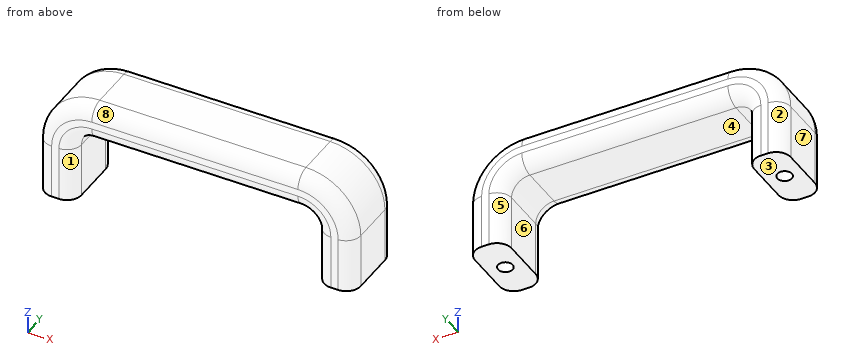
from build123d import *

# Parameters (mm, degrees)
F1_DEPTH = 25.4
F2_R     = 5.08
F3_R     = 2.54
F4_DEPTH = 25.4


with BuildPart() as f1:
    # F0 (on Front) → F1 (new body)
    with BuildSketch(Plane.XZ):
        with BuildLine():
            ThreePointArc((54.901558, 19.05), (49.321942, 32.520384), (35.851558, 38.1))
            Line((35.851558, 38.1), (-35.851558, 38.1))
            ThreePointArc((-35.851558, 38.1), (-49.321942, 32.520384), (-54.901558, 19.05))
            Line((-54.901558, 19.05), (-54.901558, 0))
            Line((-54.901558, 0), (-42.201558, 0))
            Line((-42.201558, 0), (-42.201558, 19.05))
            ThreePointArc((-42.201558, 19.05), (-40.341686, 23.540128), (-35.851558, 25.4))
            Line((-35.851558, 25.4), (35.851558, 25.4))
            ThreePointArc((35.851558, 25.4), (40.341686, 23.540128), (42.201558, 19.05))
            Line((42.201558, 19.05), (42.201558, 0))
            Line((42.201558, 0), (54.901558, 0))
            Line((54.901558, 0), (54.901558, 19.05))
        make_face()
    extrude(amount=F1_DEPTH)

    # F2
    f2_edges = [f1.edges().sort_by_distance(p)[0] for p in [
        (0, -25.4, 38.1),
        (0, 0, 38.1),
        (0, -25.4, 25.4),
        (0, 0, 25.4),
    ]]
    fillet(f2_edges, radius=F2_R)

    # F3 (on Top) → F4 (cut)
    with BuildSketch(Plane.XY):
        with Locations((-48.551558, -12.7)):
            Circle(F3_R)
        with Locations((48.551558, -12.7)):
            Circle(F3_R)
    extrude(amount=F4_DEPTH, mode=Mode.SUBTRACT)


solid = f1.part
Part model, mm, in its own coordinate system. Face numbers are marked on the shaded views. A direction names the side the tool comes from. Coordinates: 2 decimals unless noted, no trailing zeros. Loops run counter-clockwise (first coordinate to the right, second up) from the corner with the lowest first, then second, coordinate; pieces in that order, holes last. Notation, with made-up numbers: (18, 34) - (51, 34) arc R23 cw to (51, 57) - close; hole circle Ø1 at (89, 1). An arc over 180 degrees is marked (long way). Write each question's results on one line, items separated by ' | '. Start each with the question number.
Q1. Slice it at C-C on x = -5.5. Give the cut face in (y, z), and give its area (3 significant figures).
Q2. Two-plate mould, pull along X, no slides. Class the marked faces 6, 7 and 8: +X half, -X half, draft (parallel to the pull), parting line (faces both ways), or undercut.
Q3. Which spindle directions (+Z, -Z, +X, -X, +Y, -Y) get a long thin tool onto all of the face, cutting with end or side? Do the marked faces 1, 2, 3, 4 and 5. Say none if no direction does.
Q4. Slice it at B-B on y = -17.5. Give the cut face in (x, z).
Q5. Drop flat-ended pins along their axis: pin 1 Ø1 at (y, z) = (-8, 28) entering from +X; pin 2 Ø3 at (x, y) = (-48.55, -12.7) entering from +Z; pin 3 Ø6.5 at (x, y) = (48.55, -12.7) entering from -Z; pin 4 Ø6 at (y, z) = (-22.5, 24) entering from -X. Give the stop position or say it passes through.
Q6. Probe line 1 along X through (y, z) = (-13, 12); line 2 along X through (y, z) = (-9.5, 3.5); line 3 along X through (y, z) = (-11, 15). List the from-to ranges inside material, lowest first.
Q7. Slice it at D-D on y = -12.7. Give the cut face in (x, z), and give its area (3 significant figures).
Q8. Slice it at A-A on z = 18. Give the cut face in (x, y), and give its area (3 significant figures).
Answer:
1) outline: (-25.4, 30.48) arc R5.08 ccw to (-20.32, 25.4) - (-5.08, 25.4) arc R5.08 ccw to (0, 30.48) - (0, 33.02) arc R5.08 ccw to (-5.08, 38.1) - (-20.32, 38.1) arc R5.08 ccw to (-25.4, 33.02) - close | area: 300 mm2
2) face 6: undercut | face 7: -X half | face 8: draft
3) face 1: -Z, -Y | face 2: +Z, -Z, -X, +Y | face 3: -Z, +X, -X, +Y, -Y | face 4: -Z, +Y, -Y | face 5: -Z, +Y
4) outline: (-54.9, 0) - (-42.2, 0) - (-42.2, 19.05) arc R6.35 cw to (-35.85, 25.4) - (35.85, 25.4) arc R6.35 cw to (42.2, 19.05) - (42.2, 0) - (54.9, 0) - (54.9, 19.05) arc R19.05 ccw to (35.85, 38.1) - (-35.85, 38.1) arc R19.05 ccw to (-54.9, 19.05) - close
5) pin 1: stops at x = 52.92 | pin 2: stops at z = 34.46 | pin 3: stops at z = 0 | pin 4: stops at x = -54.72
6) line 1: x = -54.9 to -51.07, -46.03 to -42.2, 42.2 to 46.03, 51.07 to 54.9 | line 2: x = -54.9 to -42.2, 42.2 to 54.9 | line 3: x = -54.9 to -50.44, -46.66 to -42.2, 42.2 to 46.66, 50.44 to 54.9
7) outline: (-54.9, 0) - (-51.09, 0) - (-51.09, 25.4) - (-46.01, 25.4) - (-46.01, 0) - (-42.2, 0) - (-42.2, 19.05) arc R6.35 cw to (-35.85, 25.4) - (35.85, 25.4) arc R6.35 cw to (42.2, 19.05) - (42.2, 0) - (46.01, 0) - (46.01, 25.4) - (51.09, 25.4) - (51.09, 0) - (54.9, 0) - (54.9, 19.05) arc R19.05 ccw to (35.85, 38.1) - (-35.85, 38.1) arc R19.05 ccw to (-54.9, 19.05) - close | area: 1,640 mm2
8) outline: (-54.9, -20.32) arc R5.08 ccw to (-49.82, -25.4) - (-47.28, -25.4) arc R5.08 ccw to (-42.2, -20.32) - (-42.2, -5.08) arc R5.08 ccw to (-47.28, 0) - (-49.82, 0) arc R5.08 ccw to (-54.9, -5.08) - close; (42.2, -20.32) arc R5.08 ccw to (47.28, -25.4) - (49.82, -25.4) arc R5.08 ccw to (54.9, -20.32) - (54.9, -5.08) arc R5.08 ccw to (49.82, 0) - (47.28, 0) arc R5.08 ccw to (42.2, -5.08) - close; hole circle Ø5.08 at (-48.55, -12.7); hole circle Ø5.08 at (48.55, -12.7) | area: 560 mm2
